The model under review builds one solid part; all positions refer to its coordinate system, in mm. Give positions to 0.01 mm unless a question says otherwise; leave off trailing zeros. Loops run counter-clockwise (first coordinate to the right, second up) from the corner with the lowest first, then second, coordinate; pieces in that order, holes last. Notation, with made-up numbers: M -35.5,-9.5 L -27.5,-9.5 A22 ccw -27.5,-0.5 Z; hole C -6,34.5 d7. An arc over 180 degrees is marked long. Return JSON: item names as keys, results as strings.
```python
from build123d import *

# Parameters (mm, degrees)
F0_W     = 76.2
F0_H     = 50.8
F1_DEPTH = 1.5875
F2_R     = 2.38125
F4_DEPTH = 3.175
F3_R     = 2.38125
F5_DEPTH = 3.175


with BuildPart() as f1:
    # F0 (on Front) → F1 (new body, symmetric)
    with BuildSketch(Plane.XZ):
        Rectangle(F0_W, F0_H)
    extrude(amount=F1_DEPTH, both=True)

    # F2 (on face) → F4 (cut)
    with BuildSketch(Plane.XZ.offset(1.5875)):
        with Locations((-25.4, -6.35)):
            Circle(F2_R)
    extrude(amount=-F4_DEPTH, mode=Mode.SUBTRACT)

    # F3 (on face) → F5 (cut)
    with BuildSketch(Plane.XZ.offset(1.5875)):
        with Locations((25.4, -6.35)):
            Circle(F3_R)
    extrude(amount=-F5_DEPTH, mode=Mode.SUBTRACT)


solid = f1.part
```
1) Insertion check: pin 1 (4.5 mm diameter, centred on x = 25.4, z = -6.35, fed in from -Y) (3 decimals). The pin has a flat end and moves straight along its axis. Give the tip position at first contact, or say it passes through.
From the geometry:
{"pin 1": "through"}
2) Consider section A-A on z = -6.35. Write out the cut boundary in (x, y), then the cut area to 3 significant figures.
From the geometry:
{"outline": "M -38.1,-1.59 L -27.78,-1.59 L -27.78,1.59 L -38.1,1.59 Z; M -23.02,-1.59 L 23.02,-1.59 L 23.02,1.59 L -23.02,1.59 Z; M 27.78,-1.59 L 38.1,-1.59 L 38.1,1.59 L 27.78,1.59 Z", "area": "212 mm²"}
3) Wall thickness on L1, parallel to Z at x = 25.4, y = 0.25; L2, parallel to Z at x = 26.5, y = -0.55: over which ranges is each line inside the solid? List them lowest first. Write a range as from..to.
From the geometry:
{"L1": "-25.4..-8.73, -3.97..25.4", "L2": "-25.4..-8.46, -4.24..25.4"}
4) Consider section B-B on x = -25.4. Write out the cut boundary in (y, z).
From the geometry:
{"outline": "M -1.59,-25.4 L 1.59,-25.4 L 1.59,-8.73 L -1.59,-8.73 Z; M -1.59,-3.97 L 1.59,-3.97 L 1.59,25.4 L -1.59,25.4 Z"}
5) The part is to be moulded in two halves that separate along Z. For faces 1 (the face through (-1, -1.588, 0)), 2 (the face through (-27.78, -0.02, -6.25)), 3 (the face through (-1, 0, 25.4)), say which applies: released by +Z, released by -Z, zero draft, split by the parting line, or undercut.
From the geometry:
{"face 1": "zero draft", "face 2": "undercut", "face 3": "released by +Z"}
